Job drawing, mm, ordinate dimensions from the low corner. One solid piece. Give positions to 0.01 mm unless a question says otherwise; leave off trailing zeros. Write each loop counter-clockwise with the first axis right and the second up, starting at its lowest first coordinate (ties: lowest second). Pieces come first, ordered by that corner, then holes. Notation, with made-up numbers: (24.25, 26.5) - (52.25, 26.5) arc R21 cw to (52.25, 43.5) - close; hole circle Ø10 at (83.5, 62.5). An arc over 180 degrees is marked (long way). Answer as a JSON object with one key per item and string values.
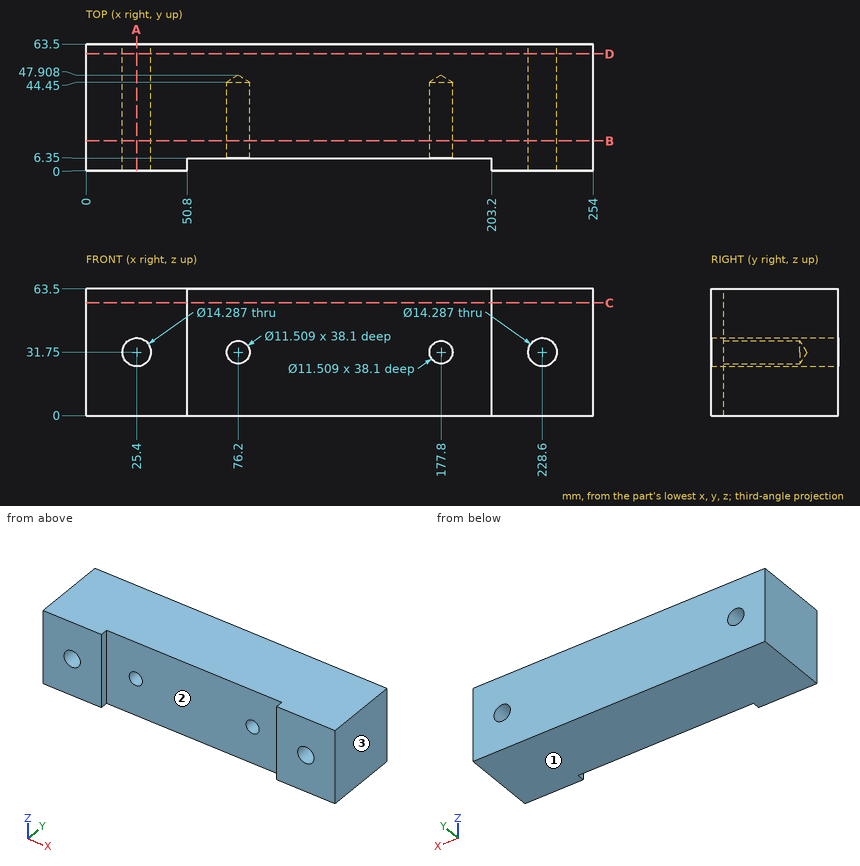
Item 1: Cut at C-C (z = 56.5). Give the cut face in (x, y).
Entries:
{"outline": "(0, 0) - (50.8, 0) - (50.8, 6.35) - (203.2, 6.35) - (203.2, 0) - (254, 0) - (254, 63.5) - (0, 63.5) - close"}
Item 2: Probe line 1 (X direction, y = 18, z = 31) (1 decimal); line 2 (X direction, y = 6, z = 54); line 3 (Z direction, x = 76.2, y = 18) (1 decimal). List the from-to ranges inside material, lowest first. Write a range as from..to.
Entries:
{"line 1": "0..18.3, 32.5..70.5, 81.9..172.1, 183.5..221.5, 235.7..254", "line 2": "0..50.8, 203.2..254", "line 3": "0..26, 37.5..63.5"}
Item 3: Flat gauge pins, fed straight in: P1, Ø1, axis at x = 197.5, z = 40, coming from the -Y side; P2, Ø13, axis at x = 25.4, z = 31.75, coming from the +Y side. Where does each tip first touch, or does it go through?
Entries:
{"P1": "y = 6.35", "P2": "through"}
Item 4: Cut at B-B (y = 15). State how many separate pieces and enclosed holes the cut face has, and give its area (3 significant figures).
Entries:
{"separate pieces": "1", "enclosed holes": "4", "area": "15,600 mm2"}
Item 5: Mould opens along X. For the marked faces 1, 2 and 3 say: +X half, -X half, draft (parallel to the pull), parting line (faces both ways), or undercut.
Entries:
{"face 1": "draft", "face 2": "undercut", "face 3": "+X half"}
Item 6: Cut at A-A (x = 25.4). Give the cut face in (y, z).
Entries:
{"outline": "(0, 0) - (63.5, 0) - (63.5, 24.61) - (0, 24.61) - close; (0, 38.89) - (63.5, 38.89) - (63.5, 63.5) - (0, 63.5) - close"}
Item 7: Cut at D-D (y = 58.5). Give the cut face in (x, z), and give its area (3 significant figures).
Entries:
{"outline": "(0, 0) - (254, 0) - (254, 63.5) - (0, 63.5) - close; hole circle Ø14.29 at (25.4, 31.75); hole circle Ø14.29 at (228.6, 31.75)", "area": "15,800 mm2"}
